```python
from build123d import *

# Parameters (mm, degrees)
BASPROSKE_W        = 6.35
BASPROSKE_H        = 9
TOOTHCUT_DEPTH     = 15.224011389
TEETHCUTS_COUNT    = 16
TEETHCUTS_ANGLE    = 337.5
BORSKE_R           = 0.5
BORE_DEPTH         = 50.0000508
CUT_EXTRUDE1_DEPTH = 10


with BuildPart() as part:
    # BasProSke → Base-Revolve (revolve)
    with BuildSketch(Plane(origin=(0, 0, 0), x_dir=(1, 0, 0), z_dir=(0, 1, 0)), mode=Mode.PRIVATE) as base_revolve_sk:
        with Locations((3.175, 4.5)):
            Rectangle(BASPROSKE_W, BASPROSKE_H)
    revolve(base_revolve_sk.sketch.rotate(Axis((-10, 0, 0), (1, 0, 0)), 180), axis=Axis((-10, 0, 0), (1, 0, 0)))

    # TooCutSke → ToothCut (cut, through all)
    with BuildSketch(Plane(origin=(0, 0, 0), x_dir=(0, 0, -1), z_dir=(1, 0, 0))):
        with BuildLine():
            ThreePointArc((0.523792937, 6.728643397), (0, 6.749), (-0.523792937, 6.728643397))
            ThreePointArc((-0.523792937, 6.728643397), (-0.828704482, 7.90962059), (-1.553355277, 8.890721711))
            ThreePointArc((-1.553355277, 8.890721711), (0, 9.0254), (1.553355277, 8.890721711))
            ThreePointArc((1.553355277, 8.890721711), (0.828704482, 7.90962059), (0.523792937, 6.728643397))
        make_face()
    toothcut = extrude(amount=TOOTHCUT_DEPTH, mode=Mode.SUBTRACT)

    # TeethCuts: ToothCut ×16 about axis
    teethcuts_axis = Axis((-10, 0, 0), (1, 0, 0))
    for i in range(1, TEETHCUTS_COUNT):
        add(toothcut.rotate(teethcuts_axis, i * TEETHCUTS_ANGLE / (TEETHCUTS_COUNT - 1)), mode=Mode.SUBTRACT)

    # BorSke → Bore (cut, symmetric)
    with BuildSketch(Plane(origin=(0, 0, 0), x_dir=(0, 0, -1), z_dir=(1, 0, 0))):
        with Locations(Location((0, 0, 0), (0, 0, 180))):
            Circle(BORSKE_R)
    extrude(amount=BORE_DEPTH, both=True, mode=Mode.SUBTRACT)

    # Sketch1 → Cut-Extrude1 (cut)
    with BuildSketch(Plane(origin=(6.35, 0, 0), x_dir=(0, 0, -1), z_dir=(1, 0, 0))):
        with BuildLine():
            ThreePointArc((0.824891111, 2.044891111), (0, 2.205), (-0.824891111, 2.044891111))
            Line((-0.824891111, 2.044891111), (-0.824891111, 0.824891111))
            Line((-0.824891111, 0.824891111), (-2.044891111, 0.824891111))
            ThreePointArc((-2.044891111, 0.824891111), (-2.205, 0), (-2.044891111, -0.824891111))
            Line((-2.044891111, -0.824891111), (-0.824891111, -0.824891111))
            Line((-0.824891111, -0.824891111), (-0.824891111, -2.044891111))
            ThreePointArc((-0.824891111, -2.044891111), (0, -2.205), (0.824891111, -2.044891111))
            Line((0.824891111, -2.044891111), (0.824891111, -0.824891111))
            Line((0.824891111, -0.824891111), (2.044891111, -0.824891111))
            ThreePointArc((2.044891111, -0.824891111), (2.164602723, -0.420142893), (2.205, 0))
            ThreePointArc((2.205, 0), (2.164602723, 0.420142893), (2.044891111, 0.824891111))
            Line((2.044891111, 0.824891111), (0.824891111, 0.824891111))
            Line((0.824891111, 0.824891111), (0.824891111, 2.044891111))
        make_face()
    extrude(amount=-CUT_EXTRUDE1_DEPTH, mode=Mode.SUBTRACT)


solid = part.part
```
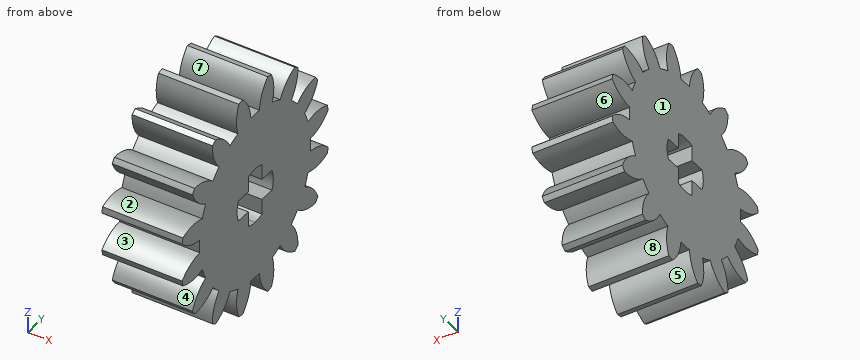
The listing builds one solid part. Answer for the finished solid, in the listing's coordinates (mm). Face numbers are marked on the shaded views. A direction names the side the tool comes from. Round coordinates to 2 decimals unless told otherwise and drop trailing zeros. Write each loop counter-clockwise with the first axis right and the second up, starting at its lowest first coordinate (ties: lowest second). Pieces come first, ordered by that corner, then holes. Notation, with made-up numbers: (48.5, 36) -> (77.5, 36) arc R23 ccw to (77.5, 71) -> close; hole circle Ø7 at (59.5, 81). An arc over 180 degrees is marked (long way). Answer as a JSON object with one key per item and string values. Group by question number.
Q1. Each of these flat-tipped pins is pushed along its axis until it touches: pin 1 Ø0.6 at (x, z) = (3.5, -1) entering from -Y; pin 2 Ø1.5 at (x, z) = (3.5, 0) entering from +Y; pin 3 Ø3 at (x, z) = (2.5, 0) entering from +Y. Where does it stop, or does it pass through?
Q2. Section B-B (y = 5.75) is taken. Write down the section's boundary in (x, z).
Q3. Straight lines are drawn through the part: line 1 along Y through (x, z) = (2, -7.5); line 2 along Y through (x, z) = (1.75, -7); line 3 along Y through (x, z) = (6.25, -6.5). For each, find the intervals that lie inside material, in ascending order.
Q4. Section A-A (z = 3.75) is taken. Write down the section's boundary in (x, y), plus the area to 3 significant figures.
Q5. Determine the mould class of the marked faces 1, 2 and 3 for opening direction Y: pulls with the +Y half, pulls with the -Y half, needs draft (parallel to the pull), parting line crosses it, or undercut.
Q6. Which of the six approach directions +Z, -Z, +X, -X, +Y, -Y give full straight-line access (tool end or side, diameter ignored) to the marked faces 4, 5, 6, 7 and 8?
Check values:
{
 "1": {"pin 1": "y = -8.63", "pin 2": "y = 7.73", "pin 3": "y = 8.84"},
 "2": {"outline": "(0, -4.82) -> (6.35, -4.82) -> (6.35, 4.82) -> (0, 4.82) -> close"},
 "3": {"line 1": "-4.97 to -4.55, -2.27 to -0.67, 0.67 to 2.27, 4.55 to 4.97", "line 2": "-5.18 to -3.8, -2.23 to -0.55, 0.55 to 2.23, 3.8 to 5.18", "line 3": "-5.1 to -3.35, -2.12 to 2.12, 3.35 to 5.1"},
 "4": {"outline": "(0, -6.95) -> (6.35, -6.95) -> (6.35, 6.95) -> (0, 6.95) -> close", "area": "88.3 mm^2"},
 "5": {"face 1": "needs draft", "face 2": "undercut", "face 3": "pulls with the -Y half"},
 "6": {"face 4": "+X, -X, -Y", "face 5": "-Z, +X, -X", "face 6": "+X, -X, +Y", "face 7": "+Z, +X, -X", "face 8": "+X, -X"}
}
